Geometry: final body of the model. Coordinates: model frame, mm. Give positions to 0.01 mm unless a question says otherwise; leave off trailing zeros. Order: outer loops, then holes, each group sorted by start corner. A loop starts at its lowest first (then second) coordinate and runs counter-clockwise, first axis right, second up. Notation, with made-up numbers: (60, 18.25) -> (91, 18.25) arc R15 ccw to (91, 30.25) -> close; hole circle Ø7 at (54, 55). An arc over 180 degrees is marked (long way). Answer in a Markdown table with one row per item. Add a question column.
Q1. Cut plane C-C on z = 1.25. Count the separate pieces of the cut face and the enclosed holes in it, and give its area (3 significant figures).
Q2. Cut plane A-A on x = -11. Return the cut outline in (y, z).
Q3. Cut plane B-B on y = 20. Return the cut outline in (x, z), and give its area (3 significant figures).
Q4. Line query: line 1 along Y through (x, z) = (165, 1.05); line 2 along X through (y, z) = (34.5, 2.25); line 3 along Y through (x, z) = (-194, 1.6). Output: solid intervals per line, ascending. Write a range as from..to.
from build123d import *

# Parameters (mm, degrees)
SKETCH1_W           = 458
SKETCH1_H           = 245
BOSS_EXTRUDE1_DEPTH = 3
CUT_EXTRUDE1_DEPTH  = 260.723410574
SKETCH3_R           = 2.5
CUT_EXTRUDE2_DEPTH  = 260.723410574
SKETCH4_W           = 428
SKETCH4_H           = 29
CUT_EXTRUDE3_DEPTH  = 260.723410574


with BuildPart() as part:
    # Sketch1 → Boss-Extrude1 (new body)
    with BuildSketch(Plane.XY):
        Rectangle(SKETCH1_W, SKETCH1_H)
    extrude(amount=BOSS_EXTRUDE1_DEPTH)

    # Sketch2 → Cut-Extrude1 (cut, through all)
    with BuildSketch(Plane.XY.offset(3)):
        with BuildLine():
            Line((-148, -107.5), (-148, -122.5))
            ThreePointArc((-148, -122.5), (-155, -129.5), (-162, -122.5))
            Line((-162, -122.5), (-162, -107.5))
            ThreePointArc((-162, -107.5), (-155, -100.5), (-148, -107.5))
        make_face()
        with BuildLine():
            Line((162, -107.5), (162, -122.5))
            ThreePointArc((162, -122.5), (155, -129.5), (148, -122.5))
            Line((148, -122.5), (148, -107.5))
            ThreePointArc((148, -107.5), (155, -100.5), (162, -107.5))
        make_face()
    extrude(amount=-CUT_EXTRUDE1_DEPTH, mode=Mode.SUBTRACT)

    # Sketch3 → Cut-Extrude2 (cut, through all)
    with BuildSketch(Plane.XY.offset(3)):
        with Locations((-194, 112.5)):
            Circle(SKETCH3_R)
        with Locations((-194, -107.5)):
            Circle(SKETCH3_R)
        with Locations((194, -107.5)):
            Circle(SKETCH3_R)
        with Locations((194, 112.5)):
            Circle(SKETCH3_R)
        with Locations((-215, 0)):
            Circle(SKETCH3_R)
        with Locations((-215, -90)):
            Circle(SKETCH3_R)
        with Locations((-215, 90)):
            Circle(SKETCH3_R)
        with Locations((215, 0)):
            Circle(SKETCH3_R)
        with Locations((215, -90)):
            Circle(SKETCH3_R)
        with Locations((215, 90)):
            Circle(SKETCH3_R)
        with Locations((0, 112.5)):
            Circle(SKETCH3_R)
        with Locations((0, -107.5)):
            Circle(SKETCH3_R)
    extrude(amount=-CUT_EXTRUDE2_DEPTH, mode=Mode.SUBTRACT)

    # Sketch4 → Cut-Extrude3 (cut, through all)
    with BuildSketch(Plane.XY.offset(3)):
        with Locations((0, 27.5)):
            Rectangle(SKETCH4_W, SKETCH4_H)
    extrude(amount=-CUT_EXTRUDE3_DEPTH, mode=Mode.SUBTRACT)


solid = part.part
Completed:
| question | item | result |
|---|---|---|
| 1 | separate pieces | 1 |
| 1 | enclosed holes | 13 |
| 1 | area | 99,000 mm² |
| 2 | outline | (-122.5, 0) -> (13, 0) -> (13, 3) -> (-122.5, 3) -> close; (42, 0) -> (122.5, 0) -> (122.5, 3) -> (42, 3) -> close |
| 3 | outline | (-229, 0) -> (-214, 0) -> (-214, 3) -> (-229, 3) -> close; (214, 0) -> (229, 0) -> (229, 3) -> (214, 3) -> close |
| 3 | area | 90.0 mm² |
| 4 | line 1 | y = -122.5..13, 42..122.5 |
| 4 | line 2 | x = -229..-214, 214..229 |
| 4 | line 3 | y = -122.5..-110, -105..13, 42..110, 115..122.5 |
